Read the model definition and answer for the solid it produces. Units are mm, in the model's axes. Face numbers are marked on the shaded views. Coordinates: 2 decimals unless noted, no trailing zeros. Loops run counter-clockwise (first coordinate to the right, second up) from the corner with the lowest first, then second, coordinate; pieces in that order, holes last. Notation, with made-up numbers: (-19, 80.25) -> (-1, 80.25) arc R31 ccw to (-1, 117.25) -> close; hole circle Ø9 at (-17, -19). An arc over 180 degrees is marked (long way). One line per question, with ' | ' between items. Start each with the question number.
```python
from build123d import *

# Parameters (mm, degrees)
SKETCH_1_R          = 15
EXTRUDE_1_DEPTH     = 9
CUT_EXTRUDE_1_REACH = 25.043
SKETCH_2_R          = 2.1
CUT_EXTRUDE_2_REACH = 25.043
SKETCH_3_R          = 1.6
SKETCH_4_R          = 3.5
CUT_EXTRUDE_3_DEPTH = 3
SKETCH_5_R          = 4
CHAMFER_1_SIZE      = 5
FILLET_2_R          = 1


with BuildPart() as part:
    # 草图1 → 凸台-拉伸1 (new body)
    with BuildSketch(Plane(origin=(0, 0, 0), x_dir=(1, 0, 0), z_dir=(0, 1, 0))):
        with Locations(Location((0, 0, 0), (0, 0, 270))):
            Circle(SKETCH_1_R)
    extrude(amount=EXTRUDE_1_DEPTH)

    # 草图2 → 切除-拉伸1 (cut, up to next)
    with BuildSketch(Plane(origin=(0, 9, 0), x_dir=(1, 0, 0), z_dir=(0, 1, 0)), mode=Mode.PRIVATE) as cut_extrude_1_sk1:
        with Locations(Location((0, 0, 0), (0, 0, 270))):
            Circle(SKETCH_2_R)
    cut_extrude_1_tool1 = extrude(cut_extrude_1_sk1.sketch, amount=-CUT_EXTRUDE_1_REACH, mode=Mode.PRIVATE) & part.part
    add(cut_extrude_1_tool1.solids().sort_by_distance((0, 9, 0))[0], mode=Mode.SUBTRACT)

    # 草图3 → 切除-拉伸2 (cut, up to next)
    with BuildSketch(Plane(origin=(0, 9, 0), x_dir=(1, 0, 0), z_dir=(0, 1, 0)), mode=Mode.PRIVATE) as cut_extrude_2_sk1:
        with Locations(Location((-6, 0, 0), (0, 0, 270))):
            Circle(SKETCH_3_R)
    cut_extrude_2_tool1 = extrude(cut_extrude_2_sk1.sketch, amount=-CUT_EXTRUDE_2_REACH, mode=Mode.PRIVATE) & part.part
    # 草图3 → 切除-拉伸2 (cut, up to next)
    with BuildSketch(Plane(origin=(0, 9, 0), x_dir=(1, 0, 0), z_dir=(0, 1, 0)), mode=Mode.PRIVATE) as cut_extrude_2_sk2:
        with Locations(Location((6, 0, 0), (0, 0, 270))):
            Circle(SKETCH_3_R)
    cut_extrude_2_tool2 = extrude(cut_extrude_2_sk2.sketch, amount=-CUT_EXTRUDE_2_REACH, mode=Mode.PRIVATE) & part.part
    add(cut_extrude_2_tool1.solids().sort_by_distance((-6, 9, 0))[0], mode=Mode.SUBTRACT)
    add(cut_extrude_2_tool2.solids().sort_by_distance((6, 9, 0))[0], mode=Mode.SUBTRACT)

    # 草图4 → 切除-拉伸3 (cut)
    with BuildSketch(Plane(origin=(0, 9, 0), x_dir=(1, 0, 0), z_dir=(0, 1, 0))):
        with Locations(Location((-6, 0, 0), (0, 0, 270))):
            Circle(SKETCH_4_R)
        with Locations(Location((6, 0, 0), (0, 0, 270))):
            Circle(SKETCH_4_R)
    extrude(amount=-CUT_EXTRUDE_3_DEPTH, mode=Mode.SUBTRACT)

    # 草图5 → 切除-旋转1 (revolve, cut)
    with BuildSketch(Plane.XY, mode=Mode.PRIVATE) as cut_revolve_1_sk:
        with Locations((15, 4.5)):
            Circle(SKETCH_5_R)
    revolve(cut_revolve_1_sk.sketch.rotate(Axis((0, 9, 0), (0, -1, 0)), 90), axis=Axis((0, 9, 0), (0, -1, 0)), mode=Mode.SUBTRACT)

    # 草图8 → 旋转1 (revolve)
    with BuildSketch(Plane(origin=(0, 0, 0), x_dir=(0, 0, -1), z_dir=(1, 0, 0)), mode=Mode.PRIVATE) as revolve_1_sk:
        with BuildLine():
            Line((15, 9), (15, 12.5))
            Line((15, 12.5), (21, 12.5))
            Line((21, 12.5), (21, 11))
            Line((21, 11), (11.074743567, 5.269650526))
            ThreePointArc((11.074743567, 5.269650526), (12.4582095, 7.588575894), (15, 8.5))
            Line((15, 8.5), (15, 9))
        make_face()
    revolve(revolve_1_sk.sketch.rotate(Axis((0, 14.925695769, 0), (0, -1, 0)), 180), axis=Axis((0, 14.925695769, 0), (0, -1, 0)))

    # 倒角1
    # the kernel refuses this chamfer: 5 mm, written as the material it takes off along each edge
    with BuildSketch(Plane(origin=(0, 12.5, 0), x_dir=(0, 0, 1), z_dir=(1, 0, 0))) as chamfer_1_piece_1_section:
        Polygon((15, CHAMFER_1_SIZE), (15 + CHAMFER_1_SIZE, 0), (15, 0), align=None)
    chamfer_1_piece_1 = revolve(axis=Axis((0, 12.5, 0), (0, -1, 0)), mode=Mode.PRIVATE)
    chamfer_1_piece_1 = split(chamfer_1_piece_1, bisect_by=Plane(origin=(0, 9, 0), z_dir=(0, 1, 0)), keep=Keep.TOP, mode=Mode.PRIVATE)
    add(chamfer_1_piece_1, mode=Mode.SUBTRACT)

    # 圆角1: read off the stored shape, not the designer's step
    # 圆角1 outline → 圆角1 (revolve, cut)
    with BuildSketch(Plane.XY):
        with BuildLine():
            Line((19.509414739, 10.139410198), (21, 10.139410198))
            Line((21, 10.139410198), (21, 12.5))
            ThreePointArc((21, 12.5), (20.546033561, 11.135748307), (19.509414739, 10.139410198))
        make_face()
    revolve(axis=Axis((0, 0, 0), (0, 1, 0)), mode=Mode.SUBTRACT)

    # Fillet 1 2 outline → Fillet 1 2 (revolve)
    with BuildSketch(Plane.XY):
        with BuildLine():
            Line((17.378679656, 9), (17.378679656, 9.878679656))
            ThreePointArc((17.378679656, 9.878679656), (16.40540961, 9.228361402), (15.257359313, 9))
            Line((15.257359313, 9), (17.378679656, 9))
        make_face()
    revolve(axis=Axis((0, 0, 0), (0, 1, 0)))

    # 圆角2
    fillet_2_edges = [part.edges().sort_by_distance(p)[0] for p in [
        (0, 5.269650526, -11.074743567),
    ]]
    fillet(fillet_2_edges, radius=FILLET_2_R)

    # 切除-放样1: read off the stored shape, not the designer's step
    # 切除-放样1: loft between two sections, ruled curve by curve
    loft_1_from = [
        Edge.make_bspline([(-7.08226986, 6.625453395, 0), (-7.030148744, 6.71564255, 0), (-6.960222336, 6.811326594, 0), (-6.767481895, 6.995615046, 0), (-6.643840469, 7.084318785, 0), (-6.337247234, 7.215130479, 0), (-6.153397528, 7.255952208, 0), (-5.761468115, 7.242597799, 0), (-5.554924915, 7.186512093, 0), (-5.194168295, 6.978027628, 0), (-5.04245146, 6.827071668, 0), (-4.835200327, 6.494154302, 0), (-4.778778635, 6.31447759, 0), (-4.739045515, 5.98352081, 0), (-4.754171349, 5.832104943, 0), (-4.817616618, 5.57309566, 0), (-4.865609023, 5.46473576, 0), (-4.969851256, 5.28435745, 0), (-5.039777664, 5.188673406, 0), (-5.232518105, 5.004384954, 0), (-5.356159531, 4.915681215, 0), (-5.662752766, 4.784869521, 0), (-5.846602472, 4.744047792, 0), (-6.238531885, 4.757402201, 0), (-6.445075085, 4.813487907, 0), (-6.805831705, 5.021972372, 0), (-6.95754854, 5.172928332, 0), (-7.164799673, 5.505845698, 0), (-7.221221365, 5.68552241, 0), (-7.260954485, 6.01647919, 0), (-7.245828651, 6.167895057, 0), (-7.182383382, 6.42690434, 0), (-7.134390977, 6.53526424, 0), (-7.08226986, 6.625453395, 0)], [0, 0, 0, 0, 0.0625, 0.0625, 0.125, 0.125, 0.1875, 0.1875, 0.25, 0.25, 0.3125, 0.3125, 0.375, 0.375, 0.4375, 0.4375, 0.5, 0.5, 0.5625, 0.5625, 0.625, 0.625, 0.6875, 0.6875, 0.75, 0.75, 0.8125, 0.8125, 0.875, 0.875, 0.9375, 0.9375, 1, 1, 1, 1], 3),
    ]
    loft_1_to = [
        Edge.make_bspline([(-11.314005718, 3.776543732, -11), (-11.374293741, 3.886044208, -11), (-11.429176294, 4.017242171, -11), (-11.498850196, 4.329564997, -11), (-11.513230125, 4.511601305, -11), (-11.457326547, 4.907675528, -11), (-11.385164779, 5.121837485, -11), (-11.128234017, 5.516096119, -11), (-10.942457221, 5.693429674, -11), (-10.504455315, 5.934581763, -11), (-10.25526136, 5.996731425, -11), (-9.784714907, 6.003002212, -11), (-9.565158312, 5.949452554, -11), (-9.20058006, 5.784884337, -11), (-9.054449158, 5.675386577, -11), (-8.827795373, 5.44949266, -11), (-8.746282304, 5.332956745, -11), (-8.625706259, 5.113955792, -11), (-8.570823706, 4.982757829, -11), (-8.501149804, 4.670435003, -11), (-8.486769875, 4.488398695, -11), (-8.542673453, 4.092324472, -11), (-8.614835221, 3.878162515, -11), (-8.871765983, 3.483903881, -11), (-9.057542779, 3.306570326, -11), (-9.495544685, 3.065418237, -11), (-9.74473864, 3.003268575, -11), (-10.215285093, 2.996997788, -11), (-10.434841688, 3.050547446, -11), (-10.79941994, 3.215115663, -11), (-10.945550842, 3.324613423, -11), (-11.172204627, 3.55050734, -11), (-11.253717696, 3.667043255, -11), (-11.314005718, 3.776543732, -11)], [0, 0, 0, 0, 0.0625, 0.0625, 0.125, 0.125, 0.1875, 0.1875, 0.25, 0.25, 0.3125, 0.3125, 0.375, 0.375, 0.4375, 0.4375, 0.5, 0.5, 0.5625, 0.5625, 0.625, 0.625, 0.6875, 0.6875, 0.75, 0.75, 0.8125, 0.8125, 0.875, 0.875, 0.9375, 0.9375, 1, 1, 1, 1], 3),
    ]
    loft_1 = Solid(Shell([*[Face.make_surface_from_curves(loft_1_from[k], loft_1_to[k]) for k in range(1)], Face(Wire(loft_1_from)), Face(Wire(loft_1_to))]))
    add(loft_1, mode=Mode.SUBTRACT)


solid = part.part
```
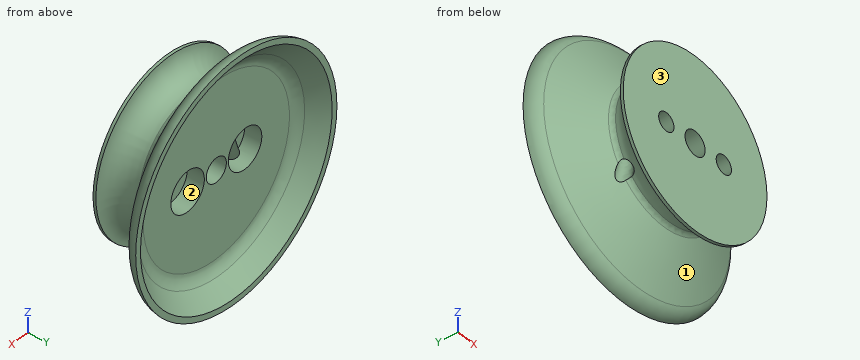
(1) Section B-B on y = 8.5 is taken. Write down the section's boundary in (x, z), plus the area to 3 significant figures.
(2) Section A-A on z = 1 is taken. Give the number of separate pieces and of enclosed holes in the cut face, plus the area to 3 significant figures.
(3) Section C-C on y = 10.75 is taken. Write down the section's boundary in (x, z), plus the area to 3 significant figures.
(4) Find the intervals of material crossed by probe 1 along X at (y, z) = (7.7, 0); probe 2 along X at (y, z) = (3.75, 0); probe 3 along Z at (x, y) = (6.5, 11), in increasing order. Write a range as from..to.
(5) Determine the mould class of the marked faces 1, 2 and 3 for opening direction Z: +Z half, -Z half, draft (parallel to the pull), parting line (faces both ways), or undercut.
(6) Each of these flat-tipped pins is pushed along its axis until it touches: pin 1 Ø2.5 at (x, z) = (0, 0) entering from +Y; pin 2 Ø15.5 at (x, z) = (-5.5, -4) entering from +Y; pin 3 Ø5.5 at (x, z) = (-6.5, -0.5) entering from +Y; pin 4 Ø5 at (y, z) = (5, -2) entering from +X. Where does it stop, or does it pass through?
Working result:
1) outline: circle Ø33.34 at (0, 0); hole circle Ø7 at (-6, 0); hole circle Ø4.2 at (0, 0); hole circle Ø7 at (6, 0) | area: 782 mm2
2) separate pieces: 4 | enclosed holes: 0 | area: 141 mm2
3) outline: circle Ø40.51 at (0, 0); hole circle Ø36.5 at (0, 0) | area: 243 mm2
4) probe 1: x = -15.28..-9.5, -2.5..-2.1, 2.1..2.5, 9.5..15.28 | probe 2: x = -11.07..-7.6, -4.4..-2.1, 2.1..4.4, 7.6..11.07 | probe 3: z = -19.39..-17.32, 17.32..19.39
5) face 1: parting line | face 2: undercut | face 3: draft
6) pin 1: passes through | pin 2: stops at y = 9 | pin 3: stops at y = 6 | pin 4: stops at x = 14.82
